Geometry check sheet. Reference: the model listing, model coordinates, mm. Face numbers are marked on the shaded views. A direction names the side the tool comes from. Coordinates: 2 decimals unless noted, no trailing zeros. Loops run counter-clockwise (first coordinate to the right, second up) from the corner with the lowest first, then second, coordinate; pieces in that order, holes last. Notation, with made-up numbers: (47, 4.5) - (62, 4.5) arc R18 ccw to (62, 25.5) - close; hole circle Ø1 at (53.25, 13.5). An arc over 180 degrees is marked (long way). One line per item, written item: value.
from build123d import *

# Parameters (mm, degrees)
SKETCH1_W           = 180
SKETCH1_H           = 20
BOSS_EXTRUDE2_DEPTH = 1
BOSS_EXTRUDE3_DEPTH = 1
BOSS_EXTRUDE5_START = 1
BOSS_EXTRUDE5_DEPTH = 1
SKETCH6_W           = 182
SKETCH6_H           = 70
BOSS_EXTRUDE6_DEPTH = 1
FILLET2_R           = 0.2


with BuildPart() as part:
    # Sketch1 → Boss-Extrude2 (new body)
    with BuildSketch(Plane(origin=(0, 0, 0), x_dir=(1, 0, 0), z_dir=(0, 1, 0))):
        with Locations((0, 10)):
            Rectangle(SKETCH1_W, SKETCH1_H)
    extrude(amount=BOSS_EXTRUDE2_DEPTH)

    # Sketch3 → Boss-Extrude3 (add)
    with BuildSketch(Plane(origin=(90, 0, 0), x_dir=(0, 0, -1), z_dir=(1, 0, 0))):
        with BuildLine():
            Line((0, 1), (0, -69))
            Line((0, -69), (100, -69))
            Line((100, -69), (100, -64.892848271))
            ThreePointArc((100, -64.892848271), (71.821490362, -17.594043661), (20, 1))
            Line((20, 1), (0, 1))
        make_face()
    extrude(amount=BOSS_EXTRUDE3_DEPTH)

    # Sketch5 → Boss-Extrude5 (add)
    with BuildSketch(Plane.ZY.offset(90).offset(BOSS_EXTRUDE5_START)):
        with BuildLine():
            Line((0, 1), (-20, 1))
            ThreePointArc((-20, 1), (-71.821490362, -17.594043661), (-100, -64.892848271))
            Line((-100, -64.892848271), (-100, -69))
            Line((-100, -69), (0, -69))
            Line((0, -69), (0, 1))
        make_face()
    extrude(amount=-BOSS_EXTRUDE5_DEPTH)

    # Sketch6 → Boss-Extrude6 (add)
    with BuildSketch(Plane.XY):
        with Locations((0, -34)):
            Rectangle(SKETCH6_W, SKETCH6_H)
    extrude(amount=BOSS_EXTRUDE6_DEPTH)

    # Fillet2
    fillet2_edges = [part.edges().sort_by_distance(p)[0] for p in [
        (91, 1, -9.5),
        (91, -17.594043661, -71.821490362),
        (-91, 1, -9.5),
        (-91, -17.594043661, -71.821490362),
        (-91, -34, 1),
        (91, -34, 1),
        (0, 1, 1),
    ]]
    fillet(fillet2_edges, radius=FILLET2_R)


solid = part.part
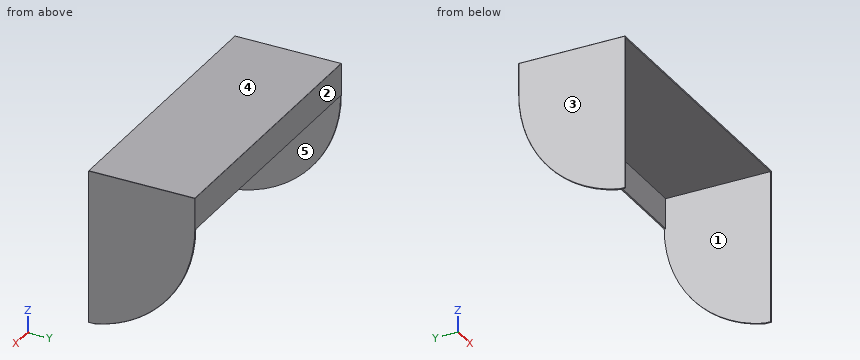
(1) Material ranges on probe 1 along X at (y, z) = (-29, -64.5); probe 2 along Y at (x, z) = (70.5, -14.5), recorded low to high. Write a range as from..to.
Reply:
probe 1: -91..-90, 90..91
probe 2: 0..1
(2) Go/stop test with flat-tipped pins: pin 1 Ø1.1 at (x, y) = (40, 0.5) entering from -Z; pin 2 Ø10 at (x, z) = (29.5, -14) entering from -Y. Record where each tip stops, or that it passes through.
Reply:
pin 1: z = -20
pin 2: y = 0
(3) Release check for a two-part mould opening along X. For the marked faces 1, 2 and 3 record: pulls with the +X half, pulls with the -X half, needs draft (parallel to the pull), parting line crosses it, or undercut.
Reply:
face 1: undercut
face 2: needs draft
face 3: pulls with the -X half
(4) Cross-section at A-A on x = -13. Record the cut outline in (y, z).
Reply:
outline: (-69, 0) - (0, 0) - (0, -20) - (1, -20) - (1, 0.8) arc R0.2 ccw to (0.8, 1) - (-69, 1) - close
(5) Access from +Z, -Z, +X, -X, +Y, -Y to the whole of each face (thin tool, end or side, straight path). Record for the marked faces 4 and 5.
Reply:
face 4: +Z, +X, -X, +Y, -Y
face 5: -Z, -Y
